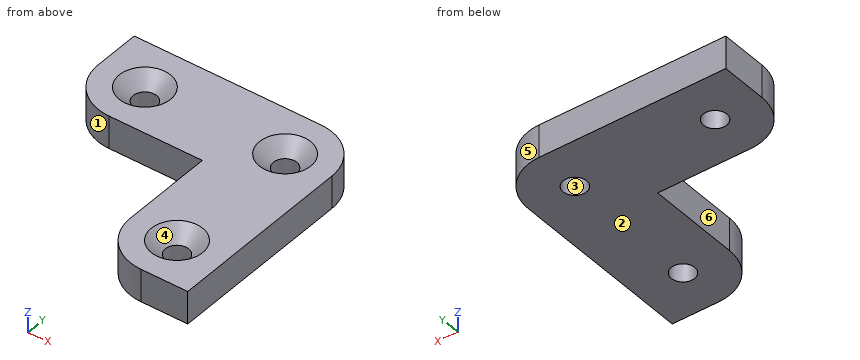
```python
from build123d import *

# Parameters (mm, degrees)
F0_R     = 2.5
F1_DEPTH = 7
F2_R     = 10
F3_SIZE  = 3


# Not quite as in the source:
# - a feature names something its author has since deleted; it is built from what else it names


with BuildPart() as f1:
    # F0 (on Top) → F1 (new body)
    with BuildSketch(Plane.XY):
        Polygon((0, -50), (0, 0), (-50, 0), (-50, -20), (-20, -20), (-20, -50), align=None)
        with Locations((-10, -40)):
            Circle(F0_R, mode=Mode.SUBTRACT)
        with Locations((-40, -10)):
            Circle(F0_R, mode=Mode.SUBTRACT)
        with Locations((-10, -10)):
            Circle(F0_R, mode=Mode.SUBTRACT)
    extrude(amount=F1_DEPTH)

    # F2
    f2_edges = [f1.edges().sort_by_distance(p)[0] for p in [
        (0, 0, 3.5),
        (-20, -50, 3.5),
        (-50, -20, 3.5),
    ]]
    fillet(f2_edges, radius=F2_R)

    # F3
    f3_edges = [f1.edges().sort_by_distance(p)[0] for p in [
        (-42.5, -10, 7),
        (-12.5, -40, 7),
        (-12.5, -10, 7),
    ]]
    chamfer(f3_edges, length=F3_SIZE)


solid = f1.part
```
Build history of the part. All positions in model axes, mm. Face numbers are marked on the shaded views. A direction names the side the tool comes from. Coordinates: 2 decimals unless noted, no trailing zeros. Write each loop counter-clockwise with the first axis right and the second up, starting at its lowest first coordinate (ties: lowest second). Pieces come first, ordered by that corner, then holes.
1. Pull direction Y, two halves, no side cores. Call the marked faces 1, 2, 3 and 4: released by +Y, released by -Y, zero draft, split by the parting line, or undercut.
Answer block:
face 1: released by -Y
face 2: zero draft
face 3: undercut
face 4: undercut
2. Band-saw the part on B-B, the plane x = -11.5. Give the number of separate pieces and of enclosed holes in the cut face, and give its area (3 significant figures).
Answer block:
separate pieces: 3
enclosed holes: 0
area: 273 mm2
3. Band-saw the part on C-C, the plane x = -33. Give the cut face in (y, z).
Answer block:
outline: (-20, 0) - (0, 0) - (0, 7) - (-20, 7) - close
4. 3-axis set-ups, long thin cutter, end or side, ignore diameter. For the marked faces 5 and 6: which of +Z, -Z, +X, -X, +Y, -Y reach the whole face in a straight line?
Answer block:
face 5: +Z, -Z, +X, +Y
face 6: +Z, -Z, -X, -Y
5. Band-saw the part on D-D, the plane x = -19. Give the cut face in (y, z), and give its area (3 significant figures).
Answer block:
outline: (-44.36, 0) - (0, 0) - (0, 7) - (-44.36, 7) - close
area: 311 mm2
6. Band-saw the part on A-A, the plane z = 5.75. Give the cut face in (x, y), and give its area (3 significant figures).
Answer block:
outline: (-50, -10) arc R10 ccw to (-40, -20) - (-20, -20) - (-20, -40) arc R10 ccw to (-10, -50) - (0, -50) - (0, -10) arc R10 ccw to (-10, 0) - (-50, 0) - close; hole circle Ø8.5 at (-40, -10); hole circle Ø8.5 at (-10, -40); hole circle Ø8.5 at (-10, -10)
area: 1,370 mm2
7. Drill centre lines: probe 1 along X at (y, z) = (-10.5, 6.75); probe 2 along Y at (x, z) = (-40, 1); probe 3 along Y at (x, z) = (-9.5, 4.5). Where is each one in solid material? Low to high.
Answer block:
probe 1: x = -49.99 to -45.23, -34.77 to -15.23, -4.77 to 0
probe 2: y = -20 to -12.5, -7.5 to 0
probe 3: y = -50 to -42.96, -37.04 to -12.96, -7.04 to -0.01
8. Drop flat-ended pins along their axis: pin 1 (2 mm diameter, centred on y = -8, z = 3, fed in from +X); pin 2 (4 mm diameter, centred on x = -10, y = -40, fed in from -Z); pin 3 (6 mm diameter, centred on x = -10, y = -10, fed in from +Z); pin 4 (1.5 mm diameter, centred on x = -24.5, z = 2.5, fed in from -Y). Give the stop position or say it passes through.
Answer block:
pin 1: stops at x = -0.05
pin 2: passes through
pin 3: stops at z = 4.5
pin 4: stops at y = -20
